Autodesk Inventor part; units mm, degrees
ref_plane "Work Plane11" through (-14.3169, 0, -30.2866) normal (-0.0053, 0.9986, 0.0521) x (0.9949, 0, 0.1013)
ref_plane "YZ Plane" through (0, 0, 0) normal (1, 0, 0) x (0, 1, 0)
ref_plane "XY Plane" through (0, 0, 0) normal (0, 0, 1) x (1, 0, 0)
sketch "Sketch1" plane through (0, 0, 0) normal (0, 1, 0) x (-1, 0, 0)
  circle A0 centre (0, 0) radius 10
  line L0 (10, 0) -> (9.2097, -30.1236) construction
  arc A1 (-17.027, -27.0939) -> (14.3169, -30.2866) centre (17.8178, 159.5407) ccw construction
  line L1 (0, 0) -> (-14.0737, -27.6212) construction
  line L2 (10, 0) -> (-10, 0) construction
  line L3 (0, -10) -> (0, 10) construction
  arc A2 (9.7489, -2.227) -> (9.2097, -30.1236) centre (76.4766, -17.4702) ccw
  arc A3 (-14.0737, -27.6212) -> (-9.4804, -3.1816) centre (-33.645, -11.2914) ccw
  line L4 (0, 0) -> (9.2097, -30.1236) construction
  line L5 (14.3169, -30.2866) -> (-17.027, -27.0939) construction
  line L6 (9.2097, -30.1236) -> (-14.0737, -27.6212) construction
  line L7 (-1.355, -28.6902) -> (-1.4214, -29.3415) construction
  line L8 (0, 0) -> (-17.027, -27.0939) construction
  line L9 (0, 0) -> (14.3169, -30.2866) construction
  line L10 (-17.027, -27.0939) -> (-14.0737, -27.6212) construction
  line L11 (0, 0) -> (-18.5691, -57.0543) construction
  line L12 (0, 0) -> (17.8587, -58.3272) construction
  line L13 (17.8587, -58.3272) -> (-18.5691, -57.0543) construction
  line L14 (-18.5691, -57.0543) -> (-17.027, -27.0939) construction
  line L15 (14.3169, -30.2866) -> (17.8587, -58.3272) construction
  line L16 (14.3169, -30.2866) -> (17.8587, -58.3272) construction
  line L17 (-17.027, -27.0939) -> (-18.5691, -57.0543) construction
  line L18 (17.8587, -58.3272) -> (31.4475, -86.1902) construction
  line L19 (-18.5691, -57.0543) -> (3.1581, -110.8309) construction
  line L20 (-18.5691, -57.0543) -> (39.4309, -57.0543) construction
  arc A4 (17.8587, -58.3272) -> (31.4475, -86.1902) centre (65.5771, -52.3) ccw construction
  arc A5 (-18.5691, -57.0543) -> (3.1581, -110.8309) centre (50.0978, -60.5886) ccw construction
  line L21 (31.4475, -86.1902) -> (3.1581, -110.8309) construction
  arc A6 (-14.0737, -27.6212) -> (9.2097, -30.1236) centre (17.8178, 159.5407) ccw
  dimension "d0" = 20
  dimension "d4" = 63
  dimension "d7" = 31
  dimension "d8" = 73
  dimension "d9" = 31.5
  dimension "d14" = 32
  dimension "d15" = 33.5
  dimension "d19" = 3
  dimension "d20" = 60
  dimension "d21" = 61
  dimension "d22" = 36.45
  dimension "d23" = 30
  dimension "d24" = 68.4466
  dimension "d25" = 25.4892
  dimension "d26" = 118
  dimension "d27" = 31
  dimension "d28" = 58
  dimension "d29" = 68
  dimension "d30" = 37.5161
  dimension "d142" = 28.2635
  dimension "d149" = 87.13
  dimension "d150" = 103.015
  dimension "d152" = 65.999
ref_plane "Work Plane11" through (-14.3169, 0, -30.2866) normal (-0.0053, 0.9986, 0.0521) x (0.9949, 0, 0.1013)
sketch "Sketch9" plane through (-14.3169, 0, -30.2866) normal (-0.0053, 0.9986, 0.0521) x (0.9949, 0, 0.1013)
  line L0 (0, 0) -> (31.5061, 0)
  line L1 (31.5061, 0) -> (30.004, 29.9624)
  line L2 (0, 0) -> (-6.3652, 27.5369)
  line L3 (-6.3652, 27.5369) -> (30.004, 29.9624) construction
  line L4 (-6.3652, 27.5369) -> (-22.7067, 53.88)
  line L5 (-22.7067, 53.88) -> (2.9398, 81.2608)
  line L6 (2.9398, 81.2608) -> (30.004, 29.9624)
  point P0 (17.3123, -28.6406)
  dimension "d141" = 30
  dimension "d143" = 28.263
  dimension "d144" = 36.45
  dimension "d146" = 58
  dimension "d147" = 31
  dimension "d148" = 37.516
  dimension "d151" = 87.13
  dimension "d153" = 66
extrude "Extrusion6" add sketch "Sketch1" along normal mid plane 4.5
extrude "Extrusion7" add sketch "Sketch9" along normal mid plane 10
properties part number "brace2.0"
Geometry check sheet. Reference: the model listing, model coordinates, mm. Coordinates: 2 decimals unless noted, no trailing zeros. Loops run counter-clockwise (first coordinate to the right, second up) from the corner with the lowest first, then second, coordinate; pieces in that order, holes last. Notation, with made-up numbers: (64.5, 54.25) - (77.5, 54.25) arc R29 cw to (77.5, 82.25) - close; hole circle Ø11 at (-33, -0.75). An arc over 180 degrees is marked (long way). One line per item, written item: value. Start each with the question number.
(1) Mould release check, pull along Z, two halves, no side actions. Record for faces 1 (the cylindrical face through (-8.04, -0.03, -16.22)), 2 (the flat face through (-1, -2.25, -10)): released by +Z, released by -Z, zero draft, split by the parting line, or undercut.
(2) Material ranges on line 1 (Y direction, x = -3, z = -23.5); line 2 (Y direction, x = -17, z = -60.5); line 3 (X direction, y = 5.75, z = -70.5), recorded low to high. Write a range as [from, to].
(3) Cross-section at B-B on z = 0. Enter the section's corners in (x, y).
(4) Cross-section at C-C on x = -23.5. Enter the section's corners in (y, z), plus the area to 3 significant figures.
(5) Cross-section at A-A on x = 0. Enter the section's corners in (y, z).
(6) Depth check by flat-ended pin: P1, Ø6, axis at x = -9.5, z = -40.5, coming from the -Y side; P2, Ø1.5, axis at y = 4.5, z = -77.5, coming from the -X side; P3, Ø1, axis at x = -0.5, z = -92, coming from the -Y side. Enter the tip coordinate at first touch or a pass-through.
Results below:
1. face 1: undercut
1. face 2: zero draft
2. line 1: y = [-2.25, 2.25]
2. line 2: y = [-3.44, 6.57]
2. line 3: x = [-23.94, 13.01]
3. outline: (-10, -2.25) - (10, -2.25) - (10, 2.25) - (-10, 2.25) - close
4. outline: (-2.98, -70.14) - (-1.77, -93.27) - (8.22, -92.8) - (7, -69.51) - close
4. area: 232 mm2
5. outline: (-4.99, -29.09) - (-1.13, -103.21) - (8.85, -102.56) - (4.99, -28.57) - (2.25, -28.71) - (2.25, 10) - (-2.25, 10) - (-2.25, -28.95) - close
6. P1: stops at y = -4.61
6. P2: stops at x = -27.68
6. P3: stops at y = -1.74
